Autodesk Inventor part; units mm, degrees
ref_plane "YZ Plane" through (0, 0, 0) normal (1, 0, 0) x (0, 1, 0)
ref_plane "XZ Plane" through (0, 0, 0) normal (0, 1, 0) x (-1, 0, 0)
ref_plane "XY Plane" through (0, 0, 0) normal (0, 0, 1) x (1, 0, 0)
sketch "Skizze1" plane through (0, 0, 0) normal (0, 0, 1) x (1, 0, 0)
  line L0 (-273, 285) -> (68, 285)
  line L1 (68, -8) -> (-273, -8)
  line L2 (5, 153.9294) -> (5, 157.0706)
  line L3 (5, 253.9294) -> (5, 257.0706)
  line L4 (0, 285) -> (-235, 285)
  line L5 (-235, 285) -> (-235, -8)
  line L6 (-235, -8) -> (0, -8)
  line L7 (0, -8) -> (0, 285)
  line L8 (-199.0415, -3.8) -> (-199.0415, -6)
  line L9 (-138, 2) -> (-138, 4.5)
  line L10 (-250, 282.9) -> (-250, -5.9)
  point P0 (0, 0)
  point P1 (-273, -8)
  dimension "d0" = 5
  dimension "d1" = 0
  dimension "d2" = 0
  dimension "d15" = 15
extrude "Grobblech1" add sketch "Skizze1" along normal blind 2
sketch "Skizze2" plane through (-235, -6, 2) normal (0, -1, 0) x (1, 0, 0)
  line L0 (235, 0) -> (0, 0)
  line L1 (0, 0) -> (0, -18)
  line L2 (0, -18) -> (235, -18)
  line L3 (235, -18) -> (235, 0)
edge flange "Lasche1" height 18 angle 90 thickness 2 bend radius 2 thickness toward (0, -1, 0) relief tear relief width 2 relief depth 1 corner gap 2 corner form 0 edges at (-117.5, -8, 0) (-117.5, 285, 0) wall of the first edge with corners at (0, -6, 2) (-235, -6, 2) (-235, -6, -16) (0, -6, -16)
bend "Biegung1"
corner "Ecke1"
sketch "Skizze3" plane through (0, 0, 2) normal (0, 0, 1) x (1, 0, 0)
  line L0 (-273, 285) -> (68, 285) construction
  line L1 (0, 281) -> (0, -4) construction
  line L2 (0, 281) -> (0, 285) construction
  line L3 (0, -8) -> (0, -4) construction
  line L4 (68, -8) -> (-273, -8) construction
  line L5 (-235, -4) -> (-235, 281) construction
  line L6 (-235, 285) -> (-235, 281) construction
  line L7 (-235, -4) -> (-235, -8) construction
  line L8 (-250, 282.9) -> (-250, -5.9) construction
  line L9 (-225, 285) -> (-225, -8) construction
  line L10 (0, -8) -> (-235, -8)
  line L11 (-225, 285) -> (-217, 285)
  line L12 (-217, 285) -> (-217, -8)
  line L13 (-217, -8) -> (-225, -8)
  line L14 (-225, -8) -> (-225, 285)
  point P0 (0, 0)
  dimension "d16" = 25
  dimension "d17" = 8
  dimension "d18" = 293
extrude "Extrusion1" cut sketch "Skizze3" against normal blind 4.75
equation "\"d4\" = Stärke"
equation "\"d5\" = BreiteBiegungsfreistellung"
equation "\"d6\" = TiefeBiegungsfreistellung"
equation "\"d7\" = MinimalRest"
equation "\"d8\" = Übergangsradius"
equation "\"d11\" = Biegeradius"
equation "\"d12\" = GrößeEckenfreistellung"
equation "\"d13\" = Abstandsgröße"
equation "\"d14\" = JacobiRadiusGröße"
equation "\"Biegeradius\" = Stärke"
equation "\"BreiteBiegungsfreistellung\" = Stärke"
equation "\"TiefeBiegungsfreistellung\" = 0.5 * Stärke"
equation "\"GrößeEckenfreistellung\" = 4 * Stärke"
equation "\"MinimalRest\" = 2 * Stärke"
equation "\"Übergangsradius\" = Biegeradius"
equation "\"JacobiRadiusGröße\" = Biegeradius"
equation "\"Abstandsgröße\" = Stärke"
properties part number "EinschubRechts"
Input: part model. Units: mm. Frame: model coordinates. A direction names the side the tool comes from. Coordinates: 2 decimals unless noted, no trailing zeros. Loops run counter-clockwise (first coordinate to the right, second up) from the corner with the lowest first, then second, coordinate; pieces in that order, holes last.
Q1. Section B-B, the plane z = -12.25. Return the cut outline in (x, y), and give its area (3 significant figures).
Results are:
outline: (-235, -8) - (0, -8) - (0, -6) - (-235, -6) - close; (-235, 283) - (0, 283) - (0, 285) - (-235, 285) - close
area: 940 mm2
Q2. Line query: line 1 along Y through (x, z) = (-159.5, -7.5); line 2 along X through (y, z) = (195, 1); line 3 along Z through (x, y) = (-17.5, 258). Output: solid intervals per line, ascending.
Results are:
line 1: y = -8 to -6, 283 to 285
line 2: x = -235 to -225, -217 to 0
line 3: z = 0 to 2
Q3. Set-up query: faces 1 (the flat face through (-119, -6, -9)), 2 (the flat face through (-110, 140, 2)). Return all of +Z, -Z, +X, -X, +Y, -Y with unobstructed straight access to the full face (end or side cutting, diameter ignored); none if empty.
Results are:
face 1: -Z, +X, -X
face 2: +Z, +X, -X, +Y, -Y
Q4. Section C-C, the plane x = -46.5. Return the cut outline in (y, z), and give its area (3 significant figures).
Results are:
outline: (-8, -16) - (-6, -16) - (-6, -2) arc R2 cw to (-4, 0) - (281, 0) arc R2 cw to (283, -2) - (283, -16) - (285, -16) - (285, -2) arc R4 ccw to (281, 2) - (-4, 2) arc R4 ccw to (-8, -2) - close
area: 645 mm2
Q5. Mould query, pull axis Y, two halves, no side actions, for faces 3 (the flat face through (-119, -8, -9)), 4 (the flat face through (-116, 283, -9)), 5 (the flat face through (0, 138, 1)), 6 (the flat face through (-110, 140, 0)). Classes: +Y half, -Y half, draft (parallel to the pull), parting line (faces both ways), or undercut.
Results are:
face 3: -Y half
face 4: undercut
face 5: draft
face 6: undercut
Q6. Contact query for flat-ended pins moving along their axis: pin 1 (11 mm diameter, centred on x = -230, y = 131.5, fed in from -Z); pin 2 (2 mm diameter, centred on x = -219.5, y = 283.5, fed in from +Z); pin 3 (8 mm diameter, centred on x = -94.5, z = -1, fed in from +Y). Output: stop coordinate, or through.
Results are:
pin 1: stops at z = 0
pin 2: stops at z = -2.75
pin 3: stops at y = 285
Q7. Section A-A, the plane y = 121. Return the cut outline in (x, z), and give its area (3 significant figures).
Results are:
outline: (-235, 0) - (-225, 0) - (-225, 2) - (-235, 2) - close; (-217, 0) - (0, 0) - (0, 2) - (-217, 2) - close
area: 454 mm2
